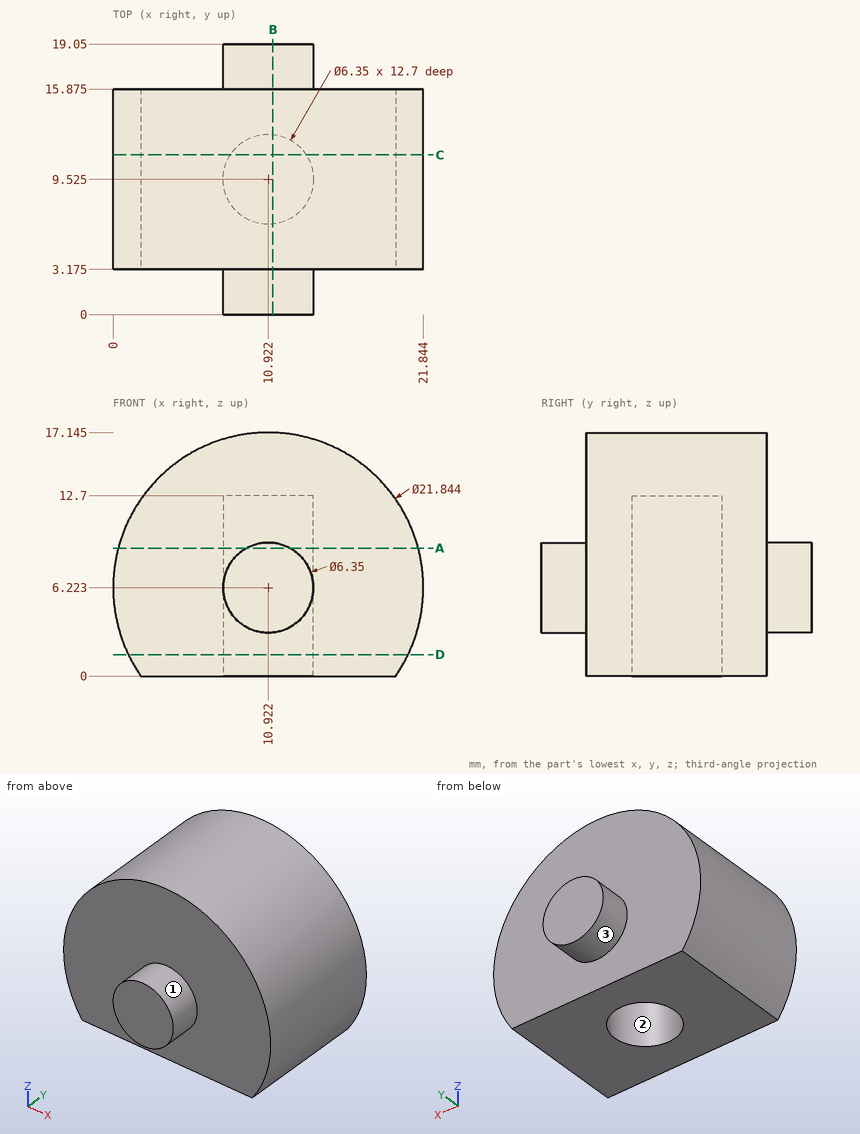
Input: dimensioned drawing with shaded views. Units: mm. Origin: part minimum x, y, z. A direction names the side the tool comes from. Coordinates: 2 decimals unless noted, no trailing zeros. Order: outer loops, then holes, each group sorted by start corner. A loop starts at its lowest first (then second) coordinate and runs counter-clockwise, first axis right, second up.
1. Cut plane D-D, the plane z = 1.5. Return loops of the section in (x, y) (3 decimals), plus the area to 3 significant figures.
Checked values:
outline: (1.074, 3.175) - (20.77, 3.175) - (20.77, 15.875) - (1.074, 15.875) - close; hole circle Ø6.35 at (10.922, 9.525)
area: 218 mm2
2. Ray query, line 1 along Y through (x, z) = (2.5, 6.5) (3 decimals); line 2 along Z through (x, y) = (10.75, 6.5); line 3 along X through (y, z) = (10.25, 9). Return the intervals inside material, ascending.
Checked values:
line 1: y = 3.175 to 15.875
line 2: z = 12.7 to 17.14
line 3: x = 0.36 to 7.83, 14.01 to 21.49
3. Cut plane A-A, the plane z = 9. Return loops of the section in (x, y) (3 decimals), plus the area to 3 significant figures.
Checked values:
outline: (0.359, 3.175) - (9.383, 3.175) - (9.383, 0) - (12.461, 0) - (12.461, 3.175) - (21.485, 3.175) - (21.485, 15.875) - (12.461, 15.875) - (12.461, 19.05) - (9.383, 19.05) - (9.383, 15.875) - (0.359, 15.875) - close; hole circle Ø6.35 at (10.922, 9.525)
area: 256 mm2
4. Cut plane C-C, the plane y = 11.25. Return loops of the section in (x, z).
Checked values:
outline: (1.95, 0) - (8.26, 0) - (8.26, 12.7) - (13.59, 12.7) - (13.59, 0) - (19.9, 0) arc R10.92 ccw (long way) to start
5. Access query for the marked faces 1, 2 and 3. Directions: +Z, -Z, +X, -X, +Y, -Y. A direction counts if a zero-diameter tool reaches every point of the face in a straight line with its end or side. Return the directions, or none.
Checked values:
face 1: -Y
face 2: -Z
face 3: +Y
6. Cut plane B-B, the plane x = 11.25. Return loops of the section in (y, z) (3 decimals), plus the area to 3 significant figures.
Checked values:
outline: (0, 3.065) - (3.175, 3.065) - (3.175, 0) - (6.367, 0) - (6.367, 12.7) - (12.683, 12.7) - (12.683, 0) - (15.875, 0) - (15.875, 3.065) - (19.05, 3.065) - (19.05, 9.381) - (15.875, 9.381) - (15.875, 17.14) - (3.175, 17.14) - (3.175, 9.381) - (0, 9.381) - close
area: 178 mm2
7. Contact query for flat-ended pins moving along their axis: P1, Ø1, axis at y = 11, z = 11.5, coming from the +X side; P2, Ø1.5, axis at x = 17, z = 11.5, coming from the +Y side (3 decimals); P3, Ø10, axis at y = 13, z = 14.5, coming from the -X side. Output: stop coordinate, or through.
Checked values:
P1: stops at x = 20.74
P2: stops at y = 15.875
P3: stops at x = 0.5
